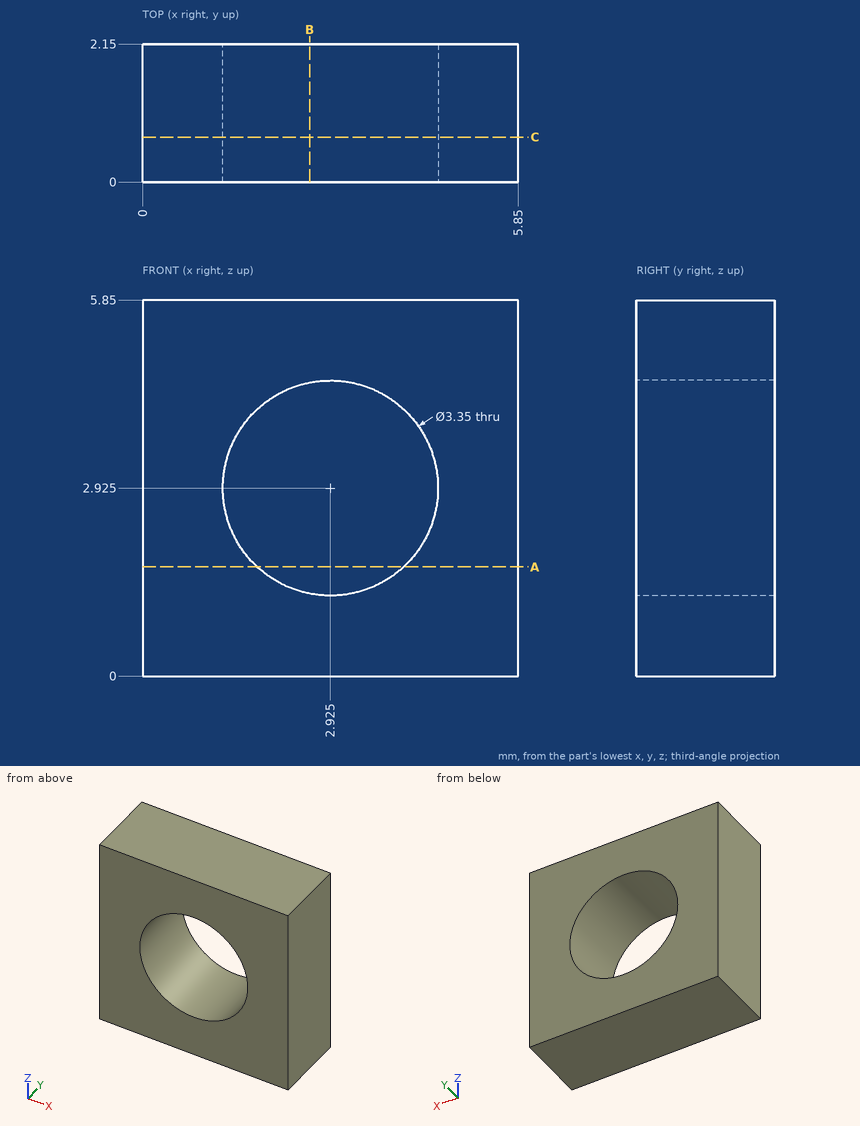
The drawing under review shows one solid part. Ordinate dimensions are in mm from its lowest x, y, z. Give positions to 0.01 mm unless a question says otherwise; leave off trailing zeros. Write each loop counter-clockwise with the first axis right and the second up, starting at its lowest first coordinate (ties: lowest second). Pieces come first, ordered by that corner, then holes. Notation, with made-up numbers: (-2, 35) -> (18, 35) arc R33 ccw to (18, 73) -> close; hole circle Ø2 at (18.25, 42.5). An arc over 180 degrees is marked (long way). Use CSV: the item, a comma, the result in double quotes.
Q1. To check wall thickness, follow probe 1 along X at (y, z) = (0.6, 4.4); probe 2 along X at (y, z) = (0.2, 1.85); probe 3 along Z at (x, y) = (2.05, 1.55). State the ranges of each line that lie inside material, in increasing order. Write a range as [from, to].
Conclusion:
probe 1,"[0, 2.13], [3.72, 5.85]"
probe 2,"[0, 1.64], [4.21, 5.85]"
probe 3,"[0, 1.5], [4.35, 5.85]"
Q2. Take a section at A-A, the plane z = 1.7. Write out the cut boundary in (x, y), then the cut area to 3 significant figures.
Conclusion:
outline,"(0, 0) -> (1.78, 0) -> (1.78, 2.15) -> (0, 2.15) -> close; (4.07, 0) -> (5.85, 0) -> (5.85, 2.15) -> (4.07, 2.15) -> close"
area,"7.67 mm2"
Q3. Take a section at C-C, the plane y = 0.7. Write out the cut boundary in (x, z) (3 decimals), then the cut area to 3 significant figures.
Conclusion:
outline,"(0, 0) -> (5.85, 0) -> (5.85, 5.85) -> (0, 5.85) -> close; hole circle Ø3.35 at (2.925, 2.925)"
area,"25.4 mm2"
Q4. Take a section at B-B, the plane x = 2.6. Write out the cut boundary in (y, z).
Conclusion:
outline,"(0, 0) -> (2.15, 0) -> (2.15, 1.28) -> (0, 1.28) -> close; (0, 4.57) -> (2.15, 4.57) -> (2.15, 5.85) -> (0, 5.85) -> close"
Q5. For P1, Ø1, axis at x = 5, z = 1.5, coming from the -Y side, flat-tipped, find the tip position at first contact; note if it passes through.
Conclusion:
P1,"y = 0"
